Autodesk Inventor part; units mm, degrees
ref_plane "YZ Plane" through (0, 0, 0) normal (1, 0, 0) x (0, 1, 0)
ref_plane "XZ Plane" through (0, 0, 0) normal (0, 1, 0) x (-1, 0, 0)
ref_plane "XY Plane" through (0, 0, 0) normal (0, 0, 1) x (1, 0, 0)
sketch "Sketch1" plane through (0, 0, 0) normal (0, 0, 1) x (1, 0, 0)
  arc A0 (0, 25.4) -> (0, -25.4) centre (0, 0) ccw
  arc A1 (0, 31.75) -> (0, -31.75) centre (0, 0) ccw
  line L0 (0, 31.75) -> (0, 25.4)
  line L1 (0, 7.578) -> (0, -31.75)
  line L2 (0, 31.75) -> (0, 38.1)
  line L3 (0, 38.1) -> (-12.7, 38.1)
  line L4 (-12.7, 38.1) -> (-12.7, 31.75)
  line L5 (-12.7, 31.75) -> (-19.05, 31.75)
  line L6 (0, -31.75) -> (0, -38.1)
  line L7 (0, -38.1) -> (-12.7, -38.1)
  line L8 (-12.7, -38.1) -> (-12.7, -31.75)
  line L9 (-12.7, -31.75) -> (-19.05, -31.75)
  line L10 (-61.0513, 9.525) -> (-147.1395, 9.525)
  circle A2 centre (-165.1, 0) radius 12.7
  circle A3 centre (-165.1, 0) radius 15.875
  line L11 (-147.1395, -9.525) -> (-61.0513, -9.525)
  arc A4 (-19.05, -31.75) -> (-61.0513, -9.525) centre (-61.0513, -60.325) ccw
  arc A5 (-61.0513, 9.525) -> (-19.05, 31.75) centre (-61.0513, 60.325) ccw
  arc A6 (-155.1219, 12.3472) -> (-147.1395, 9.525) centre (-147.1395, 22.225) ccw
  arc A7 (-147.1395, -9.525) -> (-155.1219, -12.3472) centre (-147.1395, -22.225) ccw
  line L12 (-127, 0) -> (-50.8, 0) construction
  line L13 (-127, 6.35) -> (-50.8, 6.35)
  line L14 (-50.8, -6.35) -> (-127, -6.35)
  arc A8 (-127, 6.35) -> (-127, -6.35) centre (-127, 0) ccw
  arc A9 (-50.8, -6.35) -> (-50.8, 6.35) centre (-50.8, 0) ccw
  line L15 (0, -25.4) -> (0, -31.75)
  line L16 (0, 31.75) -> (0, 25.4)
  point P0 (-88.9, 0)
  dimension "d0" = 165.1
  dimension "d1" = 25.4
  dimension "d2" = 31.75
  dimension "d3" = 76.2
  dimension "d4" = 50.8
  dimension "d5" = 50.8
  dimension "d6" = 12.7
  dimension "d7" = 12.7
  dimension "d8" = 31.75
  dimension "d9" = 25.4
  dimension "d10" = 6.35
  dimension "d11" = 6.35
  dimension "d12" = 12.7
  dimension "d14" = 19.05
  dimension "d16" = 19.05
  dimension "d17" = 9.525
  dimension "d18" = 38.1
  dimension "d21" = 19.05
  dimension "d22" = 12.7
  dimension "d23" = 76.2
  dimension "d24" = 50.8
  dimension "d37" = 0
extrude "Extrusion1" add sketch "Sketch1" along normal mid plane 6.35 contours A0 L1 A1 L0 | A1 L6 L7 L8 L9 A4 L11 A7 A3 A6 L10 A5 L5 L4 L3 L2 | A3 | L13 A9 L14 A8
extrude "Extrusion2" add sketch "Sketch1" along normal mid plane 25.4 contours A0 L1 A1 L0 | A3
extrude "Extrusion3" add sketch "Sketch1" along normal mid plane 12.7 contours A1 L6 L7 L8 L9 A4 L11 A7 A3 A6 L10 A5 L5 L4 L3 L2
sketch "Sketch2" plane through (0, 0, 0) normal (1, 0, 0) x (0, 1, 0)
  line L0 (38.1, -6.35) -> (38.1, 6.35)
  circle A0 centre (38.1, 0) radius 3.175
  circle A1 centre (-38.1, 0) radius 3.175
  arc A2 (38.1, -6.35) -> (38.1, 6.35) centre (38.1, 0) ccw
  arc A3 (-38.1, 6.35) -> (-38.1, -6.35) centre (-38.1, 0) ccw
  line L1 (38.1, 6.35) -> (38.1, -6.35)
  line L2 (-38.1, 6.35) -> (-38.1, -6.35)
  line L3 (-38.1, -6.35) -> (-38.1, 6.35)
  point P0 (0, 0)
  dimension "d31" = 6.35
  dimension "d32" = 6.35
extrude "Extrusion4" add sketch "Sketch2" against normal blind 12.7 contours L0 A0 A2 | L0 A0 | L2 A1 | A1 L2 A3 picked at (40.0502, 0.2355) picked at (-38.971, -0.6012)
extrude "Extrusion5" cut sketch "Sketch2" against normal blind 12.7 contours A0 L0 | L0 A0 | A1 L2 | L2 A1
equation "\"d32\" = d31"
properties part number "HW 7 Part 3" material "Steel, Carbon"
Can you work these out from the model? Positions are in its coordinate system, mm. A direction names the side the tool comes from. Give positions to 0.01 mm unless a question says otherwise; leave off trailing zeros. Order: outer loops, then holes, each group sorted by start corner. A loop starts at its lowest first (then second) coordinate and runs counter-clockwise, first axis right, second up. Notation, with made-up numbers: M 11,29 L 17,29 A18 ccw 17,57 Z; hole C 51.5,-11 d10. An arc over 180 degrees is marked long. Use one line per item in the form item = value. Start each with the question number.
Item 1: If we section it at A-A (z = 0): State how many separate pieces and enclosed holes the cut face has, then the cut area to 3 significant figures.
Item 2: For faces 1 (the flat face through (-88, -6.35, 5)), 2 (the cylindrical face through (-6.26, -44.45, 0.14)), 3 (the cylindrical face through (-36.986, 15.587, -0.089)), 4 (the cylindrical face through (-37.6, -15.26, -0.09)), 5 (the cylindrical face through (-133.35, -0.14, -4.78)), which set-ups out of +Z, -Z, +X, -X, +Y, -Y let a thin tool reach every point of the face, with its end or its side?
Item 3: If I drill on line 1 along Y through (x, z) = (-96, 5.5) (3 decimals); line 2 along Y through (x, z) = (-165.1, 6.25) (3 decimals); line 3 along X through (y, z) = (-8.5, 10.25), over which ranges is the centre line in solid material (lowest first)?
Item 4: If we section it at B-B (z = 9): Write out the boundary of the cut face in (x, y) (3 decimals), then the cut area to 3 significant figures.
Item 5: We'd pull the mould along X, two halves only. Please class faces 6 (the flat face through (-89, 6.35, -5)), 7 (the cylindrical face through (-6.26, -41.27, 0.14)), 8 (the flat face through (0, 33, 0)): +X half, -X half, draft (parallel to the pull), parting line (faces both ways), or undercut.
Item 6: If we section it at D-D (x = -114): Write out the boundary of the cut face in (y, z) (3 decimals), then the cut area to 3 significant figures.
Item 7: Will these pins go through, and if not, where does the flat tip stop? pin 1 Ø14 at (y, z) = (-40, 1.5) entering from -X; pin 2 Ø4 at (x, z) = (-82.5, -6.5) entering from +Y (3 decimals); pin 3 Ø6 at (x, z) = (-152.5, -8.5) entering from +Y; pin 4 Ø5.5 at (y, z) = (38.1, 0) entering from -X.
Outcome:
q1.separate_pieces = 3
q1.enclosed_holes = 1
q1.area = 3,700 mm2
q2.face_1 = +Z
q2.face_2 = +X, -X, -Y
q2.face_3 = +Z, -Z, +Y
q2.face_4 = +Z, -Z, -Y
q2.face_5 = -Z
q3.line_1 = -9.525 to -6.35, 6.35 to 9.525
q3.line_2 = -15.875 to -12.7, 12.7 to 15.875
q3.line_3 = -178.51 to -174.54, -155.66 to -151.69, -30.59 to -23.94
q4.outline = C -165.1,0 d31.75; M 0,-31.75 L 0,-25.4 A25.4 cw 0,25.4 L 0,31.75 A31.75 ccw Z; hole C -165.1,0 d25.4
q4.area = 855 mm2
q5.face_6 = undercut
q5.face_7 = draft
q5.face_8 = +X half
q6.outline = M -9.525,-6.35 L -6.35,-6.35 L -6.35,-3.175 L 6.35,-3.175 L 6.35,-6.35 L 9.525,-6.35 L 9.525,6.35 L 6.35,6.35 L 6.35,3.175 L -6.35,3.175 L -6.35,6.35 L -9.525,6.35 Z
q6.area = 161 mm2
q7.pin_1 = -12.7
q7.pin_2 = 9.525
q7.pin_3 = 12.64
q7.pin_4 = through
